The figure shows three views and two pictorial views of one solid part (mm, origin at its lowest corner). Answer the questions. Coordinates: 2 decimals unless noted, no trailing zeros. Write each loop counter-clockwise with the first axis right and the second up, starting at its lowest first coordinate (ties: lowest second). Pieces come first, ordered by that corner, then holes. Notation, with made-up numbers: (60, 49.25) - (95, 49.25) arc R13 ccw to (95, 53.25) - close; hole circle Ø5 at (-14.5, 74.25). An arc over 180 degrees is marked (long way). Use a Markdown table: item, result. Add a question column.
(1) The part is cut by section A-A, the plane x = 16.4. Give the vertices of the cut face in (y, z).
(2) Find the intervals of material crossed by line 1 (Y direction, x = 63.6, z = 3.15); line 2 (X direction, y = 74.5, z = 5); line 3 (X direction, y = 72.5, z = 2.3) (1 decimal), in increasing order. Write a range as from..to.
(3) The part is cut by section C-C, the plane z = 3.1. Give the vertices of the cut face in (x, y).
(4) The part is cut by section B-B, the plane x = 58. Give the vertices of the cut face in (y, z).
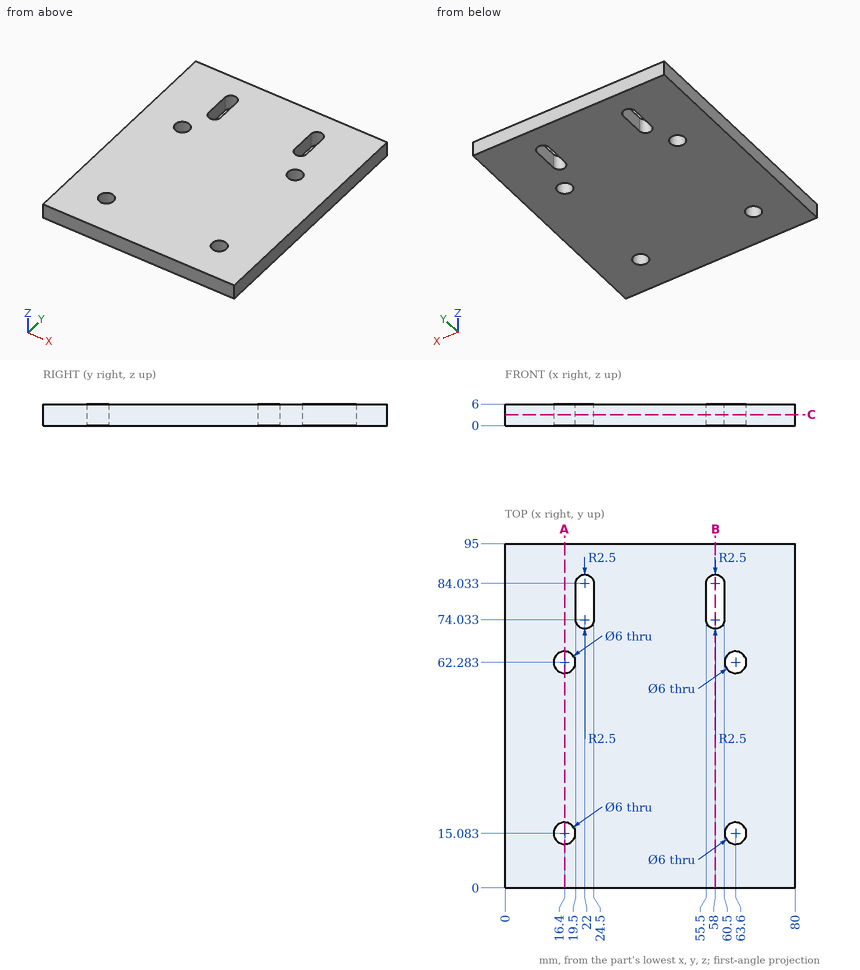
Model answer:
| question | item | result |
|---|---|---|
| 1 | outline | (0, 0) - (12.08, 0) - (12.08, 6) - (0, 6) - close; (18.08, 0) - (59.28, 0) - (59.28, 6) - (18.08, 6) - close; (65.28, 0) - (95, 0) - (95, 6) - (65.28, 6) - close |
| 2 | line 1 | 0..12.08, 18.08..59.28, 65.28..95 |
| 2 | line 2 | 0..19.5, 24.5..55.5, 60.5..80 |
| 2 | line 3 | 0..20, 24..56, 60..80 |
| 3 | outline | (0, 0) - (80, 0) - (80, 95) - (0, 95) - close; hole circle Ø6 at (16.4, 15.08); hole circle Ø6 at (16.4, 62.28); hole (19.5, 74.03) arc R2.5 ccw to (24.5, 74.03) - (24.5, 84.03) arc R2.5 ccw to (19.5, 84.03) - close; hole (55.5, 74.03) arc R2.5 ccw to (60.5, 74.03) - (60.5, 84.03) arc R2.5 ccw to (55.5, 84.03) - close; hole circle Ø6 at (63.6, 15.08); hole circle Ø6 at (63.6, 62.28) |
| 4 | outline | (0, 0) - (71.53, 0) - (71.53, 6) - (0, 6) - close; (86.53, 0) - (95, 0) - (95, 6) - (86.53, 6) - close |
